```python
from build123d import *

# Parameters (mm, degrees)
F0_W     = 31.75
F0_H     = 31.75
F0_W_2   = 25.4
F0_H_2   = 25.4
F1_DEPTH = 3.175
F2_DEPTH = 6.35
F6_R     = 3.17499


# Not quite as in the source:
# - a fillet or chamfer is up to 0.001 mm smaller than in the source, because OpenCascade refuses the exact size


with BuildPart() as f1:
    # F0 (on Top) → F1 (new body)
    with BuildSketch(Plane.XY):
        Rectangle(F0_W, F0_H)
        Rectangle(F0_W_2, F0_H_2, mode=Mode.SUBTRACT)
        Rectangle(F0_W_2, F0_H_2)
        with BuildLine():
            ThreePointArc((0, 3.175), (2.2450640303, 2.2450640303), (3.175, 0))
            ThreePointArc((3.175, 0), (2.2450640303, -2.2450640303), (0, -3.175))
            ThreePointArc((0, -3.175), (-3.175, 0), (0, 3.175))
        make_face(mode=Mode.SUBTRACT)
        with BuildLine():
            ThreePointArc((0, -3.175), (2.2450640303, -2.2450640303), (3.175, 0))
            ThreePointArc((3.175, 0), (2.2450640303, 2.2450640303), (0, 3.175))
            Line((0, 3.175), (0, -3.175))
        make_face()
        with BuildLine():
            Line((0, -3.175), (0, 3.175))
            ThreePointArc((0, 3.175), (-3.175, 0), (0, -3.175))
        make_face()
    extrude(amount=F1_DEPTH)

    # F0 (on Top) → F2 (join)
    with BuildSketch(Plane.XY):
        Rectangle(F0_W, F0_H)
        Rectangle(F0_W_2, F0_H_2, mode=Mode.SUBTRACT)
    extrude(amount=F2_DEPTH)

    # F3 (on face) → F4 (revolve)
    with BuildSketch(Plane.XY.offset(3.175)):
        with BuildLine():
            Line((0, -3.175), (0, 3.175))
            ThreePointArc((0, 3.175), (-3.175, 0), (0, -3.175))
        make_face()
    revolve(axis=Axis((0, 0, 3.175), (0, 1, 0)))

    # F0 (on Top) → F5 (revolve, cut)
    with BuildSketch(Plane.XY):
        with BuildLine():
            Line((0, -3.175), (0, 3.175))
            ThreePointArc((0, 3.175), (-3.175, 0), (0, -3.175))
        make_face()
    revolve(axis=Axis((0, 0, 0), (0, 1, 0)), mode=Mode.SUBTRACT)

    # F6 (radius 3.175 in the source; OpenCascade refuses exactly that, so slightly less here)
    f6_edges = [f1.edges().sort_by_distance(p)[0] for p in [
        (0, 12.7, 6.35),
        (12.7, 0, 6.35),
        (-12.7, 0, 6.35),
        (0, -12.7, 6.35),
    ]]
    fillet(f6_edges, radius=F6_R)


solid = f1.part
```
Geometry check sheet. Reference: the model listing, model coordinates, mm. A direction names the side the tool comes from. Coordinates: 2 decimals unless noted, no trailing zeros. Order: outer loops, then holes, each group sorted by start corner. A loop starts at its lowest first (then second) coordinate and runs counter-clockwise, first axis right, second up.
Q1. Sectioned sample at D-D on z = 1.25. Record the cut outline in (x, y) (3 decimals).
Reply:
outline: (-15.875, -15.875) - (15.875, -15.875) - (15.875, 15.875) - (-15.875, 15.875) - close; hole circle Ø5.837 at (0, 0)
Q2. Thickness scan on probe 1 along X at (y, z) = (-1, 5.75) (3 decimals); probe 2 along Y at (x, z) = (-6, 3.25) (3 decimals); probe 3 along Z at (x, y) = (-8.5, 1) (3 decimals). Record the ranges inside material, lowest first.
Reply:
probe 1: x = -15.875 to -14.018, -1.565 to 1.565, 14.018 to 15.875
probe 2: y = -15.875 to -12.701, 12.701 to 15.875
probe 3: z = 0 to 3.175
Q3. Tool access check on faces 4 (the face through (0, 4, 0)), 5 (the face through (13.61, 0.22, 5.4)). Record the directions out of +Z, -Z, +X, -X, +Y, -Y that give a thin tool (end or side, any length) a straight path to the whole face; none if there is none.
Reply:
face 4: -Z, +X, -X, +Y, -Y
face 5: +Z
Q4. Sectioned sample at A-A on z = 5. Record the cut outline in (x, y) (3 decimals).
Reply:
outline: (-15.875, -15.875) - (15.875, -15.875) - (15.875, 15.875) - (-15.875, 15.875) - close; circle Ø5.196 at (0, 0); hole (-13.277, -13.277) - (13.277, -13.277) - (13.277, 13.277) - (-13.277, 13.277) - close
Q5. Draft check along X on faces 1 (the face through (-13.61, 0.22, 5.4)), 2 (the face through (15.875, 0, 3)), 3 (the face through (0, -15.875, 3)). Enter one of: released by +X, released by -X, zero draft, split by the parting line, or undercut.
Reply:
face 1: undercut
face 2: released by +X
face 3: zero draft
